Geometry: see drawing. Coordinates: mm, zero at the bounding-box minimum. Coordinates: 2 decimals unless noted, no trailing zeros. Loops run counter-clockwise (first coordinate to the right, second up) from the corner with the lowest first, then second, coordinate; pieces in that order, holes last.
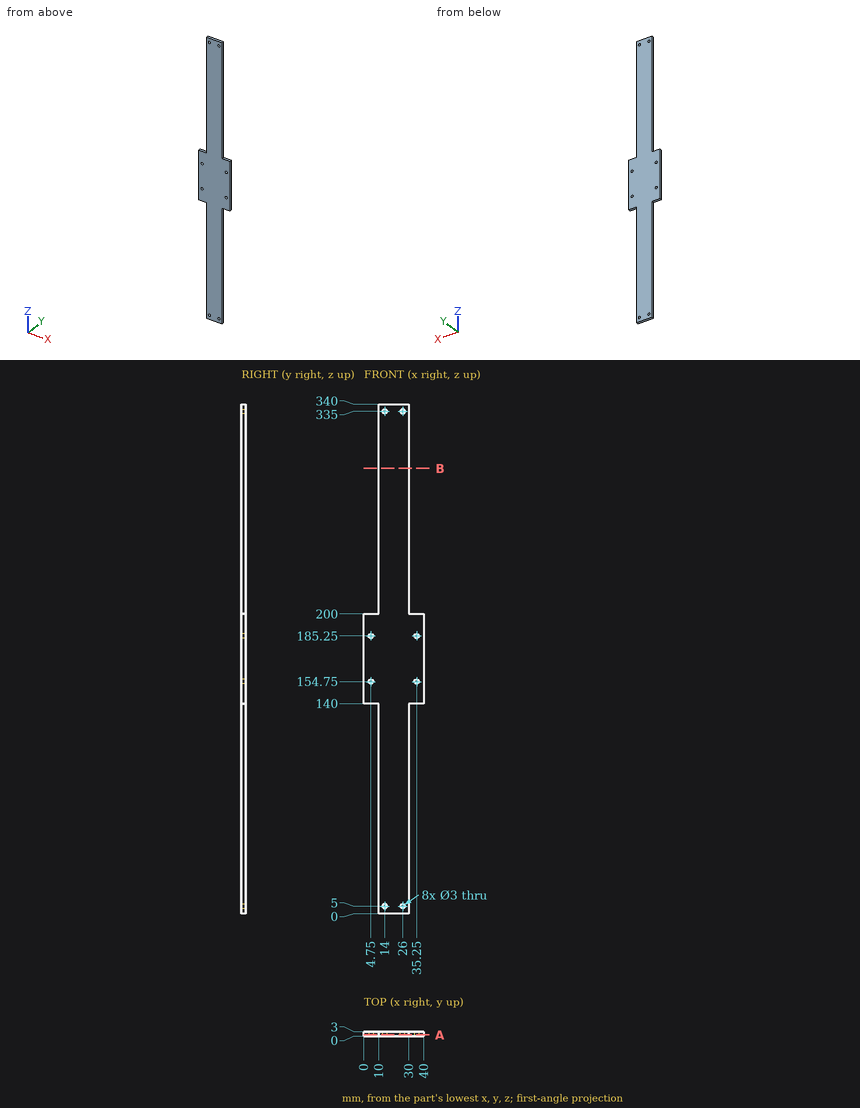
Item 1: Section query B-B (z = 297). Output: boundary loops of the cut face in (x, y), then the cut area to 3 significant figures.
Result:
outline: (10, 0) - (30, 0) - (30, 3) - (10, 3) - close
area: 60.0 mm2
Item 2: Line query: L1, parallel to X at y = 1.85, z = 5; L2, parallel to Z at x = 14, y = 1.35; L3, parallel to X at y = 2.15, z = 185.25. Output: solid intervals per line, ascending.
Result:
L1: x = 10 to 12.5, 15.5 to 24.5, 27.5 to 30
L2: z = 0 to 3.5, 6.5 to 333.5, 336.5 to 340
L3: x = 0 to 3.25, 6.25 to 33.75, 36.75 to 40
Item 3: Section query A-A (y = 0.8). Count the separate pieces of the cut face and the enclosed holes in it, then the cut area to 3 significant figures.
Result:
separate pieces: 1
enclosed holes: 8
area: 7,940 mm2
Item 4: Contact query for flat-ended pins moving along their axis: P1, Ø1, axis at x = 31.5, y = 2.5, coming from the +Z side; P2, Ø0.9, axis at x = 7.5, y = 1.5, coming from the -Z side; P3, Ø1.8, axis at x = 14, z = 335, coming from the -Y side; P4, Ø1.5, axis at y = 1, z = 295.5, coming from the +X side. Output: stop coordinate, or through.
Result:
P1: stops at z = 200
P2: stops at z = 140
P3: passes through
P4: stops at x = 30
